from build123d import *

# Parameters (mm, degrees)
SKETCH1_W           = 90
SKETCH1_H           = 100
SKETCH1_R           = 3
SKETCH1_R_2         = 3.5
BOSS_EXTRUDE1_DEPTH = 15
SKETCH2_W           = 20
SKETCH2_H           = 22
CUT_EXTRUDE1_DEPTH  = 15


with BuildPart() as part:
    # Sketch1 → Boss-Extrude1 (new body)
    with BuildSketch(Plane.XY):
        with Locations((250.418436726, 76.333548914)):
            Rectangle(SKETCH1_W, SKETCH1_H)
        with Locations((260.418436726, 76.333548914)):
            Circle(SKETCH1_R, mode=Mode.SUBTRACT)
        with Locations((240.418436726, 76.333548914)):
            Circle(SKETCH1_R, mode=Mode.SUBTRACT)
        with Locations((214.918436726, 86.833548914)):
            Circle(SKETCH1_R_2, mode=Mode.SUBTRACT)
        with Locations((214.918436726, 65.833548914)):
            Circle(SKETCH1_R_2, mode=Mode.SUBTRACT)
        with Locations((285.918436726, 86.833548914)):
            Circle(SKETCH1_R_2, mode=Mode.SUBTRACT)
        with Locations((285.918436726, 65.833548914)):
            Circle(SKETCH1_R_2, mode=Mode.SUBTRACT)
    extrude(amount=BOSS_EXTRUDE1_DEPTH)

    # Sketch2 → Cut-Extrude1 (cut)
    with BuildSketch(Plane.XY.offset(15)):
        with Locations((250.418436726, 115.333548914)):
            Rectangle(SKETCH2_W, SKETCH2_H)
    extrude(amount=-CUT_EXTRUDE1_DEPTH, mode=Mode.SUBTRACT)


solid = part.part
For this review, take the finished solid that the model builds, in its own axes (mm). A direction names the side the tool comes from. Round coordinates to 2 decimals unless told otherwise and drop trailing zeros. Loops run counter-clockwise (first coordinate to the right, second up) from the corner with the lowest first, then second, coordinate; pieces in that order, holes last. Notation, with made-up numbers: (-26, 63) - (-9, 63) arc R16 ccw to (-9, 87) - close; hole circle Ø10 at (82, -29.75). An arc over 180 degrees is marked (long way). One line per question, with ' | ' between items.
Q1. The part is to be moulded in two halves that separate along Y. For faces 1 (the flat face through (260.418, 115, 8)), 2 (the cylindrical face through (214.463, 69.304, 7.395)), 3 (the flat face through (250, 104.334, 8)), say which applies: released by +Y, released by -Y, zero draft, split by the parting line, or undercut.
Taken from the geometry:
face 1: zero draft | face 2: undercut | face 3: released by +Y
Q2. Tool access review of faces 4 (the cylindrical face through (283.141, 84.704, 7.395)), 5 (the flat face through (240.418, 115, 8)): name each direction out of +Z, -Z, +X, -X, +Y, -Y from which nothing blocks a thin tool from reaching the whole face with its end or side.
Taken from the geometry:
face 4: +Z, -Z | face 5: +Z, -Z, +Y
Q3. For pin 1 (4.5 mm diameter, centred on x = 248, z = 5.5, fed in from +Y); pin 2 (6 mm diameter, centred on x = 270.5, y = 100.5, fed in from -Z); pin 3 (5 mm diameter, centred on x = 240.42, y = 76.33, fed in from -Z), all flat-tipped, find the tip position at first contact; note any pin that passes through.
Taken from the geometry:
pin 1: stops at y = 104.33 | pin 2: stops at z = 0 | pin 3: passes through
Q4. Take a section at B-B (z = 4.5). Give the boundary of the cut face in (x, y).
Taken from the geometry:
outline: (205.42, 26.33) - (295.42, 26.33) - (295.42, 126.33) - (260.42, 126.33) - (260.42, 104.33) - (240.42, 104.33) - (240.42, 126.33) - (205.42, 126.33) - close; hole circle Ø7 at (214.92, 65.83); hole circle Ø7 at (214.92, 86.83); hole circle Ø6 at (240.42, 76.33); hole circle Ø6 at (260.42, 76.33); hole circle Ø7 at (285.92, 65.83); hole circle Ø7 at (285.92, 86.83)
Q5. For line 1 along X through (y, z) = (117, 9.75); line 2 along X through (y, z) = (75, 13.75); line 3 along Y through (x, z) = (288.5, 13.25), list the stretches that pass through material, from the lowest coordinate up. Write a range as [from, to].
Taken from the geometry:
line 1: x = [205.42, 240.42], [260.42, 295.42] | line 2: x = [205.42, 237.73], [243.11, 257.73], [263.11, 295.42] | line 3: y = [26.33, 63.47], [68.2, 84.47], [89.2, 126.33]
Q6. Take a section at A-A (x = 288). Give the boundary of the cut face in (y, z), and give its area (3 significant figures).
Taken from the geometry:
outline: (26.33, 0) - (63.02, 0) - (63.02, 15) - (26.33, 15) - close; (68.65, 0) - (84.02, 0) - (84.02, 15) - (68.65, 15) - close; (89.65, 0) - (126.33, 0) - (126.33, 15) - (89.65, 15) - close | area: 1,330 mm²
